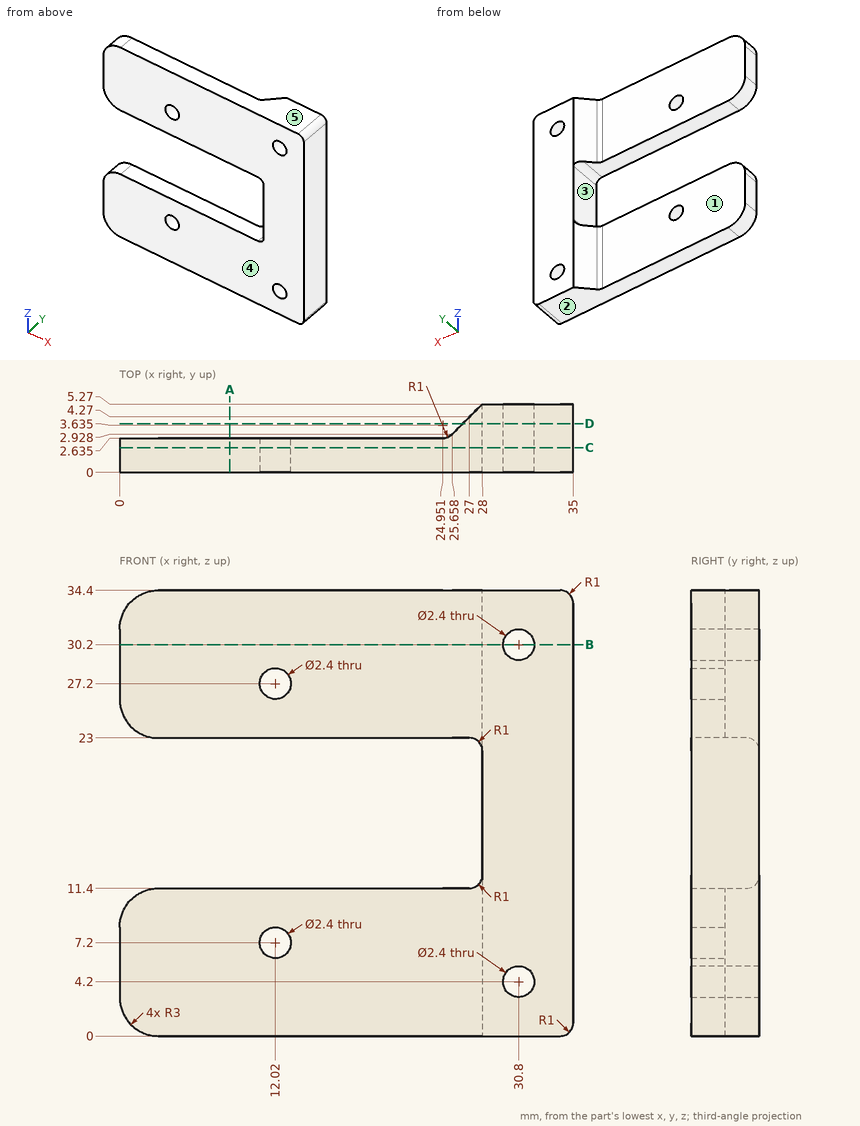
Design review of the part shown in the three views and the two pictorial views. Dimensions are in mm from the part's minimum x, y and z. A direction names the side the tool comes from. Round coordinates to 2 decimals unless told otherwise and drop trailing zeros. Loops run counter-clockwise (first coordinate to the right, second up) from the corner with the lowest first, then second, coordinate; pieces in that order, holes last. Notation, with made-up numbers: (64.25, -14.5) - (122.25, -14.5) arc R5 cw to (122.25, -5.5) - close; hole circle Ø3 at (-35, 82.25). An arc over 180 degrees is marked (long way). One line per item, written item: value. Start each with the question number.
Item 1: Take a section at B-B (z = 30.2). Give the boundary of the cut face in (x, y) (1 decimal).
Item 2: The part is to be moulded in two halves that separate along Z. For the marked faces 3, 4 and 5, say which applies: +Z half, -Z half, draft (parallel to the pull), parting line (faces both ways), or undercut.
Item 3: Take a section at D-D (y = 3.75). Give the boundary of the cut face in (x, z).
Item 4: For the marked faces 1 and 2, list the 3-axis set-ups (+Z, -Z, +X, -X, +Y, -Y) from which the entire face can be reached by the end or side of a thin tool; tool diameter is ignored.
Item 5: Clearance check with flat-ended pins moving along their axes: pin 1 Ø8 at (x, z) = (9.5, 17.5) entering from +Y; pin 2 Ø9 at (x, z) = (14.5, 27) entering from +Y (3 decimals); pin 3 Ø2.5 at (y, z) = (2.5, 18) entering from -X. State where each tip first meets the part, or that it passes through.
Item 6: Take a section at A-A (x = 8.5). Give the boundary of the cut face in (y, z) (3 decimals).
Item 7: Take a section at C-C (y = 1.9). Give the boundary of the cut face in (x, z).
Item 8: For L1, parallel to Z at x = 25.5, y = 2.5; L2, parallel to X at y = 2.2, z = 4.2; L3, parallel to Y at x = 25, z = 7.5, list the stretches that pass through material, from the lowest coordinate up.
Answer below:
1. outline: (0, 0) - (29.6, 0) - (29.6, 5.3) - (28, 5.3) - (25.7, 2.9) arc R1 cw to (25, 2.6) - (0, 2.6) - close; (32, 0) - (35, 0) - (35, 5.3) - (32, 5.3) - close
2. face 3: undercut
2. face 4: draft
2. face 5: +Z half
3. outline: (26.48, 0) - (34, 0) arc R1 ccw to (35, 1) - (35, 33.4) arc R1 ccw to (34, 34.4) - (26.48, 34.4) - (26.48, 23) - (27, 23) arc R1 cw to (28, 22) - (28, 12.4) arc R1 cw to (27, 11.4) - (26.48, 11.4) - close; hole circle Ø2.4 at (30.8, 4.2); hole circle Ø2.4 at (30.8, 30.2)
4. face 1: +Z, -Z, -X, +Y
4. face 2: -Z, +X, -X, +Y, -Y
5. pin 1: passes through
5. pin 2: stops at y = 2.635
5. pin 3: stops at x = 28
6. outline: (0, 0) - (2.635, 0) - (2.635, 11.4) - (0, 11.4) - close; (0, 23) - (2.635, 23) - (2.635, 34.4) - (0, 34.4) - close
7. outline: (0, 3) arc R3 ccw to (3, 0) - (34, 0) arc R1 ccw to (35, 1) - (35, 33.4) arc R1 ccw to (34, 34.4) - (3, 34.4) arc R3 ccw to (0, 31.4) - (0, 26) arc R3 ccw to (3, 23) - (27, 23) arc R1 cw to (28, 22) - (28, 12.4) arc R1 cw to (27, 11.4) - (3, 11.4) arc R3 ccw to (0, 8.4) - close; hole circle Ø2.4 at (12.02, 7.2); hole circle Ø2.4 at (12.02, 27.2); hole circle Ø2.4 at (30.8, 4.2); hole circle Ø2.4 at (30.8, 30.2)
8. L1: z = 0 to 11.4, 23 to 34.4
8. L2: x = 0 to 29.6, 32 to 35
8. L3: y = 0 to 2.64
